from build123d import *

# Parameters (mm, degrees)
F0_W     = 32
F0_H     = 20
F1_DEPTH = 2
F2_SIZE  = 7
F3_R     = 2.5
F4_DEPTH = 25


with BuildPart() as f1:
    # F0 (on Front) → F1 (new body)
    with BuildSketch(Plane.XZ):
        Rectangle(F0_W, F0_H)
    extrude(amount=F1_DEPTH)

    # F2
    f2_edges = [f1.edges().sort_by_distance(p)[0] for p in [
        (-16, -1, -10),
        (16, -1, -10),
    ]]
    chamfer(f2_edges, length=F2_SIZE)

    # F3 (on face) → F4 (cut)
    with BuildSketch(Plane.XZ.offset(2)):
        with BuildLine():
            ThreePointArc((-16, 2.5), (-14.232233047, 3.232233047), (-13.5, 5))
            ThreePointArc((-13.5, 5), (-14.232233047, 6.767766953), (-16, 7.5))
            Line((-16, 7.5), (-16, 2.5))
        make_face()
        with Locations((0, 5)):
            Circle(F3_R)
        with Locations((-8, -4)):
            Circle(F3_R)
        with Locations((8, -4)):
            Circle(F3_R)
        with BuildLine():
            Line((16, 2.5), (16, 7.5))
            ThreePointArc((16, 7.5), (13.5, 5), (16, 2.5))
        make_face()
    extrude(amount=-F4_DEPTH, mode=Mode.SUBTRACT)


solid = f1.part
Design review of the part built by this model. Coordinates are the model's own, in mm. Coordinates: 2 decimals unless noted, no trailing zeros. Loops run counter-clockwise (first coordinate to the right, second up) from the corner with the lowest first, then second, coordinate; pieces in that order, holes last. Notation, with made-up numbers: (22, 37) - (40, 37) arc R32 cw to (40, 75) - close; hole circle Ø2 at (77, 27.5). An arc over 180 degrees is marked (long way). Use CSV: the item, a comma, the result in double quotes. Start each with the question number.
1. Add section C-C on y = -1.2. Give the boundary of the cut face in (x, z).
2. To check wall thickness, follow probe 1 along Z at (x, y) = (-8, -0.95); probe 2 along X at (y, z) = (-0.65, -1.75); probe 3 along Z at (x, y) = (0, -1.35). State the ranges of each line that lie inside material, in increasing order.
3. Add section A-A on z = -4. Give the boundary of the cut face in (x, y).
4. Mouldability with a two-part tool opening along Z and no side actions: class faces 1 (the cylindrical face through (-9.84, -1.01, -2.31)), 2 (the flat face through (16, -1, 0)), 3 (the flat face through (13, -1, -6)) as released by +Z, released by -Z, zero draft, split by the parting line, or undercut.
5. Clearance check with a flat-ended pin moving along its axis: pin 1 (4.5 mm diameter, centred on x = 8, z = -4, fed in from +Y). State where the tip first meets the part, or that it passes through.
6. Add section D-D on z = 4.25. Give the boundary of the cut face in (x, y).
7. Add section B-B on x = -9.5. Give the boundary of the cut face in (y, z).
Resolved:
1,outline,"(-16, -3) - (-9, -10) - (9, -10) - (16, -3) - (16, 2.5) arc R2.5 cw to (16, 7.5) - (16, 10) - (-16, 10) - (-16, 7.5) arc R2.5 cw to (-16, 2.5) - close; hole circle Ø5 at (-8, -4); hole circle Ø5 at (0, 5); hole circle Ø5 at (8, -4)"
2,probe 1,"-10 to -6.5, -1.5 to 10"
2,probe 2,"-16 to -9.09, -6.91 to 6.91, 9.09 to 16"
2,probe 3,"-10 to 2.5, 7.5 to 10"
3,outline,"(-15, -2) - (-10.5, -2) - (-10.5, 0) - (-15, 0) - close; (-5.5, -2) - (5.5, -2) - (5.5, 0) - (-5.5, 0) - close; (10.5, -2) - (15, -2) - (15, 0) - (10.5, 0) - close"
4,face 1,"undercut"
4,face 2,"zero draft"
4,face 3,"released by -Z"
5,pin 1,"through"
6,outline,"(-13.62, -2) - (-2.38, -2) - (-2.38, 0) - (-13.62, 0) - close; (2.38, -2) - (13.62, -2) - (13.62, 0) - (2.38, 0) - close"
7,outline,"(-2, -9.5) - (0, -9.5) - (0, -6) - (-2, -6) - close; (-2, -2) - (0, -2) - (0, 10) - (-2, 10) - close"
